Geometry check sheet. Reference: the model listing, model coordinates, mm. A direction names the side the tool comes from. Round coordinates to 2 decimals unless told otherwise and drop trailing zeros. Write each loop counter-clockwise with the first axis right and the second up, starting at its lowest first coordinate (ties: lowest second). Pieces come first, ordered by that corner, then holes. Notation, with made-up numbers: (86, 75) -> (111, 75) arc R24 cw to (111, 85) -> close; hole circle Ø8 at (41, 77.5). An arc over 180 degrees is marked (long way). One line per question, with ' | ' between items.
Autodesk Inventor part; units mm, degrees
ref_plane "YZ Plane" through (0, 0, 0) normal (1, 0, 0) x (0, 1, 0)
ref_plane "XZ Plane" through (0, 0, 0) normal (0, 1, 0) x (-1, 0, 0)
ref_plane "XY Plane" through (0, 0, 0) normal (0, 0, 1) x (1, 0, 0)
sketch "스케치1" plane through (0, 0, 0) normal (0, 1, 0) x (-1, 0, 0)
  line L0 (0, 0) -> (24, 0)
  line L1 (24, 0) -> (24, -25)
  line L2 (24, -25) -> (0, -25)
  line L3 (0, -25) -> (0, 0)
  circle A0 centre (21.97, -2) radius 1
  circle A1 centre (2.03, -2) radius 1
  circle A2 centre (14.5, -2) radius 1
  circle A3 centre (21.97, -23) radius 1
  circle A4 centre (14.5, -23) radius 1
  circle A5 centre (2.03, -23) radius 1
  line L4 (18.75, -8.25) -> (10.25, -8.25)
  line L5 (10.25, -8.25) -> (10.25, -16.75)
  line L6 (10.25, -16.75) -> (18.75, -16.75)
  line L7 (18.75, -16.75) -> (18.75, -8.25)
  circle A6 centre (14.5, -12.5) radius 4.25
  point P0 (0, -12.5)
  point P1 (14.5, -8.25)
  point P2 (18.75, -12.5)
  point P3 (14.5, -16.75)
  point P4 (10.25, -12.5)
  dimension "d0" = 24
  dimension "d1" = 25
  dimension "d2" = 2
  dimension "d3" = 2
  dimension "d4" = 2
  dimension "d5" = 2
  dimension "d7" = 2
  dimension "d8" = 2
  dimension "d9" = 2
  dimension "d10" = 2
  dimension "d11" = 2.03
  dimension "d12" = 2.03
  dimension "d13" = 21
  dimension "d14" = 21
  dimension "d15" = 21
  dimension "d16" = 14.5
  dimension "d17" = 14.5
  dimension "d18" = 2.03
  dimension "d19" = 2.03
  dimension "d23" = 8.5
  dimension "d24" = 8.5
  dimension "d25" = 14.5
  dimension "d26" = 12.5
extrude "돌출1" add sketch "스케치1" along normal blind 1.5
extrude "돌출2" add sketch "스케치1" along normal blind 3 contours L7 A6 L4 | A6 L5 L4 | L7 L6 A6 | A6 L6 L5
extrude "돌출3" add sketch "스케치1" along normal blind 5 contours A6
properties part number "pasapery pi camera"
(1) Material ranges on line 1 (Z direction, x = -2.03, y = 0.95); line 2 (X direction, y = 0.45, z = -22.5); line 3 (Y direction, x = -0.75, z = -10.25), recorded low to high.
Resolved:
line 1: z = -25 to -24, -22 to -3, -1 to 0 | line 2: x = -24 to -22.84, -21.1 to -15.37, -13.63 to -2.9, -1.16 to 0 | line 3: y = 0 to 1.5
(2) Draft check along Z on faces 1 (the flat face through (-11, 3, -9)), 2 (the cylindrical face through (-22, 1, -22)), 3 (the flat face through (-15, 2, -8.25)). Enter one of: +Z half, -Z half, draft (parallel to the pull), parting line (faces both ways), or undercut.
Resolved:
face 1: draft | face 2: undercut | face 3: +Z half
(3) Sectioned sample at A-A on x = -21.97. Record the cut outline in (y, z).
Resolved:
outline: (0, -25) -> (1.5, -25) -> (1.5, -24) -> (0, -24) -> close; (0, -22) -> (1.5, -22) -> (1.5, -3) -> (0, -3) -> close; (0, -1) -> (1.5, -1) -> (1.5, 0) -> (0, 0) -> close
(4) Go/stop test with flat-tipped pins: pin 1 (2.5 mm diameter, centred on x = -21.97, z = -2, fed in from +Y); pin 2 (2 mm diameter, centred on y = 3.5, z = -12, fed in from -X); pin 3 (0.8 mm diameter, centred on x = -15, y = 2.5, fed in from -Z); pin 4 (1.6 mm diameter, centred on x = -2.03, z = -2, fed in from +Y). Record where each tip stops, or that it passes through.
Resolved:
pin 1: stops at y = 1.5 | pin 2: stops at x = -18.75 | pin 3: stops at z = -16.75 | pin 4: passes through
(5) Sectioned sample at B-B on z = -23. Record the cut outline in (x, y).
Resolved:
outline: (-24, 0) -> (-22.97, 0) -> (-22.97, 1.5) -> (-24, 1.5) -> close; (-20.97, 0) -> (-15.5, 0) -> (-15.5, 1.5) -> (-20.97, 1.5) -> close; (-13.5, 0) -> (-3.03, 0) -> (-3.03, 1.5) -> (-13.5, 1.5) -> close; (-1.03, 0) -> (0, 0) -> (0, 1.5) -> (-1.03, 1.5) -> close
(6) Sectioned sample at C-C on y = 0.4. Record the cut outline in (x, z), then the cut area to 3 significant figures.
Resolved:
outline: (-24, -25) -> (0, -25) -> (0, 0) -> (-24, 0) -> close; hole circle Ø2 at (-21.97, -23); hole circle Ø2 at (-21.97, -2); hole circle Ø2 at (-14.5, -23); hole circle Ø2 at (-14.5, -2); hole circle Ø2 at (-2.03, -23); hole circle Ø2 at (-2.03, -2) | area: 581 mm2
(7) Sectioned sample at D-D on z = -8.75. Record the cut outline in (x, y).
Resolved:
outline: (-24, 0) -> (0, 0) -> (0, 1.5) -> (-10.25, 1.5) -> (-10.25, 3) -> (-12.5, 3) -> (-12.5, 5) -> (-16.5, 5) -> (-16.5, 3) -> (-18.75, 3) -> (-18.75, 1.5) -> (-24, 1.5) -> close
(8) Access from +Z, -Z, +X, -X, +Y, -Y to the whole of each face (thin tool, end or side, straight path). Record for faces 4 (the cylindrical face through (-16.46, 3.99, -8.73)), 5 (the flat face through (-18.75, 2, -13)), 6 (the flat face through (-18, 3, -9)), 7 (the flat face through (-11, 3, -16)), 8 (the flat face through (-10.25, 2, -12)).
Resolved:
face 4: +Y | face 5: +Z, -Z, -X, +Y | face 6: +Z, -X, +Y | face 7: -Z, +X, +Y | face 8: +Z, -Z, +X, +Y
